Design review of the part built by this model. Coordinates are the model's own, in mm. A direction names the side the tool comes from. Round coordinates to 2 decimals unless told otherwise and drop trailing zeros. Write each loop counter-clockwise with the first axis right and the second up, starting at its lowest first coordinate (ties: lowest second). Pieces come first, ordered by that corner, then holes. Notation, with made-up numbers: (9, 61) -> (14, 61) arc R26 ccw to (14, 75) -> close; hole circle Ø1 at (-5, 18.25). An arc over 180 degrees is marked (long way). Write item = value, one per line. Start each with the question number.
Item 1: Add section A-A, the plane x = 25.4. State the section outline as (y, z) points.
Item 2: To check wall thickness, follow L1, parallel to X at y = -1, z = -25; L2, parallel to Z at x = 108.5, y = -21; L3, parallel to Z at x = 120, y = -2. State the ranges of each line that lie inside material, in increasing order.
Item 3: Add section C-C, the plane y = -32. State the section outline as (x, z) points (3 decimals).
Item 4: Mouldability with a two-part tool opening along X and no side actions: class faces 1 (the flat face through (53.975, -31, -48)), 2 (the flat face through (72, 0, -26)), 3 (the flat face through (92.075, -31, -3)), 4 (the flat face through (5.08, -15, -25)) as released by +X, released by -X, zero draft, split by the parting line, or undercut.
Item 5: Machinability: for faces 5 (the flat face through (72, -17, -5.08)), 6 (the flat face through (17, -16.51, -57)), 7 (the flat face through (143, -25.4, -27)), 8 (the flat face through (4.9, -25.4, -25.5)), 9 (the flat face through (59.69, -14, -57)), which of the approach directions +Z, -Z, +X, -X, +Y, -Y give a long, thin tool a straight path to every point of the face, cutting with its end or side? Answer none if there is none.
Item 6: For pin 1 Ø4 at (y, z) = (-29.5, -48) entering from +X (3 decimals); pin 2 Ø6.5 at (x, z) = (134, -58.5) entering from -Y; pin 3 Ø4 at (x, z) = (48, -7) entering from -Y, all flat-tipped, find the tip position at first contact; note any pin that passes through.
Item 7: Add section D-D, the plane x = 137. State the section outline as (y, z) points, then the cut area to 3 significant figures.
Item 8: Add section B-B, the plane z = -25.4. State the section outline as (x, y) points.
from build123d import *

# Parameters (mm, degrees)
SKETCH3_W           = 146.05
SKETCH3_H           = 50.8
BOSS_EXTRUDE1_DEPTH = 25.4
SHELL1_T            = -5.08
SKETCH4_R           = 12.7
CUT_EXTRUDE1_DEPTH  = 6.35
SKETCH5_W           = 19.05
SKETCH5_H           = 5.08
BOSS_EXTRUDE2_DEPTH = 11.43
SKETCH6_W           = 34.29
SKETCH6_H           = 5.08
SKETCH6_W_2         = 26.67
BOSS_EXTRUDE3_DEPTH = 12.7


with BuildPart() as part:
    # Sketch3 → Boss-Extrude1 (new body)
    with BuildSketch(Plane(origin=(0, 0, 0), x_dir=(1, 0, 0), z_dir=(0, 1, 0))):
        with Locations((73.025, 25.4)):
            Rectangle(SKETCH3_W, SKETCH3_H)
    extrude(amount=-BOSS_EXTRUDE1_DEPTH)

    # Shell1
    shell1_openings = [part.faces().sort_by_distance(p)[0] for p in [
        (73.025, -25.4, -25.4),
    ]]
    offset(amount=SHELL1_T, openings=shell1_openings, kind=Kind.INTERSECTION)

    # Sketch4 → Cut-Extrude1 (cut)
    with BuildSketch(Plane(origin=(0, 0, 0), x_dir=(1, 0, 0), z_dir=(0, 1, 0))):
        with Locations(Location((25.4, 25.4, 0), (0, 0, 270))):  # turned: the seam where the file's is
            Circle(SKETCH4_R)
        with Locations(Location((120.65, 25.4, 0), (0, 0, 270))):  # turned: the seam where the file's is
            Circle(SKETCH4_R)
    extrude(amount=-CUT_EXTRUDE1_DEPTH, mode=Mode.SUBTRACT)

    # Sketch5 → Boss-Extrude2 (add)
    with BuildSketch(Plane.XZ.offset(25.4)):
        with Locations((82.55, -2.54)):
            Rectangle(SKETCH5_W, SKETCH5_H)
        with Locations((63.5, -2.54)):
            Rectangle(SKETCH5_W, SKETCH5_H)
        with Locations((82.55, -48.26)):
            Rectangle(SKETCH5_W, SKETCH5_H)
        with Locations((63.5, -48.26)):
            Rectangle(SKETCH5_W, SKETCH5_H)
    extrude(amount=BOSS_EXTRUDE2_DEPTH)

    # Sketch6 → Boss-Extrude3 (add)
    with BuildSketch(Plane(origin=(0, 0, -50.8), x_dir=(-1, 0, 0), z_dir=(0, 0, -1))):
        with Locations((-128.905, -13.97)):
            Rectangle(SKETCH6_W, SKETCH6_H)
        with Locations((-73.025, -13.97)):
            Rectangle(SKETCH6_W_2, SKETCH6_H)
        with Locations((-17.145, -13.97)):
            Rectangle(SKETCH6_W, SKETCH6_H)
    extrude(amount=BOSS_EXTRUDE3_DEPTH)


solid = part.part
Result set:
q1.outline = (-25.4, -50.8) -> (-16.51, -50.8) -> (-16.51, -63.5) -> (-11.43, -63.5) -> (-11.43, -50.8) -> (0, -50.8) -> (0, -38.1) -> (-5.08, -38.1) -> (-5.08, -45.72) -> (-25.4, -45.72) -> close; (-25.4, -5.08) -> (-5.08, -5.08) -> (-5.08, -12.7) -> (0, -12.7) -> (0, 0) -> (-25.4, 0) -> close
q2.L1 = 0 to 12.71, 38.09 to 107.96, 133.34 to 146.05
q2.L2 = -50.8 to -45.72, -5.08 to 0
q2.L3 = -50.8 to -38.08, -12.72 to 0
q3.outline = (53.975, -50.8) -> (92.075, -50.8) -> (92.075, -45.72) -> (53.975, -45.72) -> close; (53.975, -5.08) -> (92.075, -5.08) -> (92.075, 0) -> (53.975, 0) -> close
q4.face_1 = released by -X
q4.face_2 = zero draft
q4.face_3 = released by +X
q4.face_4 = undercut
q5.face_5 = -Y
q5.face_6 = -Z, +X, -X, -Y
q5.face_7 = +Z, -Z, +X, -Y
q5.face_8 = +Z, -Z, -X, -Y
q5.face_9 = -Z, +Y, -Y
q6.pin_1 = 92.075
q6.pin_2 = -16.51
q6.pin_3 = -25.4
q7.outline = (-25.4, -50.8) -> (-16.51, -50.8) -> (-16.51, -63.5) -> (-11.43, -63.5) -> (-11.43, -50.8) -> (0, -50.8) -> (0, 0) -> (-25.4, 0) -> (-25.4, -5.08) -> (-5.08, -5.08) -> (-5.08, -45.72) -> (-25.4, -45.72) -> close
q7.area = 529 mm²
q8.outline = (0, -25.4) -> (5.08, -25.4) -> (5.08, -5.08) -> (12.7, -5.08) -> (12.7, 0) -> (0, 0) -> close; (38.1, -5.08) -> (107.95, -5.08) -> (107.95, 0) -> (38.1, 0) -> close; (133.35, -5.08) -> (140.97, -5.08) -> (140.97, -25.4) -> (146.05, -25.4) -> (146.05, 0) -> (133.35, 0) -> close
